Read the model definition and answer for the solid it produces. Units are mm, in the model's axes. Face numbers are marked on the shaded views. A direction names the side the tool comes from. Coordinates: 2 decimals unless noted, no trailing zeros. Loops run counter-clockwise (first coordinate to the right, second up) from the corner with the lowest first, then second, coordinate; pieces in that order, holes last. Notation, with made-up numbers: M -37.5,56.5 L -20.5,56.5 A34 cw -20.5,95.5 Z; hole C -35.5,69 d7. An arc over 180 degrees is marked long. One line per item, written item: value. Start each with the question number.
1. For the marked faces 1, 2, 3 and 4, determine the directions among +Z, -Z, +X, -X, +Y, -Y from which every point of the face is accessible in a straight line to the end or side of a thin tool.
2. Flat-ended cylindrical pins translate along their axes: pin 1 (6.5 mm diameter, centred on x = 98, z = 13.5, fed in from +Y); pin 2 (6.5 mm diameter, centred on y = -7, z = 27, fed in from +X); pin 3 (2 mm diameter, centred on y = -10, z = 28.5, fed in from -X). Find the tip coordinate at first contact, or state that the pin passes through.
3. The part is cut by section B-B (z = 20.3). Write down the section's boundary in (x, y), then the cut area to 3 significant figures.
4. The part is cut by section A-A (y = -13.5). Write down the section's boundary in (x, z), then the cut area to 3 significant figures.
5. Consider probe 1 along X at (y, z) = (-5.7, 20.3); probe 2 along X at (y, z) = (-7.75, 30); probe 3 along X at (y, z) = (-12.25, 17.5). Determine where each line is inside the solid, lowest interval first.
6. The part is cut by section D-D (z = 7.3). Write down the section's boundary in (x, y), then the cut area to 3 significant figures.
7. The part is cut by section C-C (x = 53). Write down the section's boundary in (y, z), then the cut area to 3 significant figures.
```python
from build123d import *

# Parameters (mm, degrees)
BOSS_EXTRUDE1_DEPTH = 40.6
SKETCH2_R           = 1.5
CUT_EXTRUDE3_DEPTH  = 24
SKETCH5_R           = 1.5
CUT_EXTRUDE4_DEPTH  = 4


with BuildPart() as part:
    # Sketch1 → Boss-Extrude1 (new body)
    with BuildSketch(Plane.XY):
        Polygon((8.125196993, -3.6), (8.125196993, -11.6), (0.125196993, -11.6), (0.125196993, -14.6), (11.125196993, -14.6), (11.125196993, -6.6), (89.125196993, -6.6), (89.125196993, -14.6), (100.125196993, -14.6), (100.125196993, -11.6), (92.125196993, -11.6), (92.125196993, -3.6), align=None)
    extrude(amount=BOSS_EXTRUDE1_DEPTH)

    # Sketch2 → Cut-Extrude3 (cut)
    with BuildSketch(Plane.XZ.offset(14.6)):
        with BuildLine():
            Line((89.125196993, 0.154767421), (89.125196993, 0))
            Line((89.125196993, 0), (100.125196993, 0))
            Line((100.125196993, 0), (100.125196993, 13))
            ThreePointArc((100.125196993, 13), (96.999405822, 4.544232737), (89.125196993, 0.154767421))
        make_face()
        with BuildLine():
            Line((89.125196993, 40.6), (89.125196993, 40.445232579))
            ThreePointArc((89.125196993, 40.445232579), (96.999405822, 36.055767263), (100.125196993, 27.6))
            Line((100.125196993, 27.6), (100.125196993, 40.6))
            Line((100.125196993, 40.6), (89.125196993, 40.6))
        make_face()
        with BuildLine():
            Line((0.125196993, 0), (11.125196993, 0))
            Line((11.125196993, 0), (11.125196993, 0.154767421))
            ThreePointArc((11.125196993, 0.154767421), (3.250988164, 4.544232737), (0.125196993, 13))
            Line((0.125196993, 13), (0.125196993, 0))
        make_face()
        with BuildLine():
            ThreePointArc((0.125196993, 27.6), (3.250988164, 36.055767263), (11.125196993, 40.445232579))
            Line((11.125196993, 40.445232579), (11.125196993, 40.6))
            Line((11.125196993, 40.6), (0.125196993, 40.6))
            Line((0.125196993, 40.6), (0.125196993, 27.6))
        make_face()
        with Locations((94.325196993, 33.3)):
            Circle(SKETCH2_R)
        with Locations((94.325196993, 7.3)):
            Circle(SKETCH2_R)
        with Locations((5.925196993, 33.3)):
            Circle(SKETCH2_R)
        with Locations((5.925196993, 7.3)):
            Circle(SKETCH2_R)
    extrude(amount=-CUT_EXTRUDE3_DEPTH, mode=Mode.SUBTRACT)

    # Sketch5 → Cut-Extrude4 (cut)
    with BuildSketch(Plane(origin=(0, -3.6, 0), x_dir=(1, 0, 0), z_dir=(0, 1, 0))):
        with Locations((25.425196993, -20.3)):
            Circle(SKETCH5_R)
        with Locations((74.825196993, -20.3)):
            Circle(SKETCH5_R)
    extrude(amount=-CUT_EXTRUDE4_DEPTH, mode=Mode.SUBTRACT)


solid = part.part
```
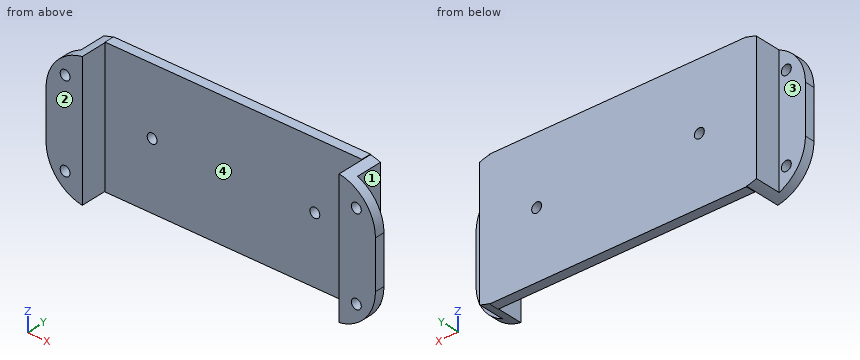
Answer block:
1. face 1: +Z, -Z, +X, +Y
1. face 2: +Z, -Z, +X, -X, -Y
1. face 3: +Z, -Z, -X, +Y
1. face 4: +Z, -Z, -Y
2. pin 1: stops at y = -11.6
2. pin 2: stops at x = 92.13
2. pin 3: stops at x = 8.13
3. outline: M 0.13,-14.6 L 11.13,-14.6 L 11.13,-6.6 L 23.93,-6.6 L 23.93,-3.6 L 8.13,-3.6 L 8.13,-11.6 L 0.13,-11.6 Z; M 26.93,-6.6 L 73.33,-6.6 L 73.33,-3.6 L 26.93,-3.6 Z; M 76.33,-6.6 L 89.13,-6.6 L 89.13,-14.6 L 100.13,-14.6 L 100.13,-11.6 L 92.13,-11.6 L 92.13,-3.6 L 76.33,-3.6 Z
3. area: 330 mm2
4. outline: M 0.13,13 A13 ccw 11.13,0.15 L 11.13,40.45 A13 ccw 0.13,27.6 Z; M 89.13,0.15 A13 ccw 100.13,13 L 100.13,27.6 A13 ccw 89.13,40.45 Z; hole C 5.93,7.3 d3; hole C 5.93,33.3 d3; hole C 94.33,7.3 d3; hole C 94.33,33.3 d3
4. area: 720 mm2
5. probe 1: x = 8.13 to 23.93, 26.93 to 73.33, 76.33 to 92.13
5. probe 2: x = 8.13 to 11.13, 89.13 to 92.13
5. probe 3: x = 0.13 to 11.13, 89.13 to 100.13
6. outline: M 1.44,-14.6 L 4.43,-14.6 L 4.43,-11.6 L 1.44,-11.6 Z; M 7.43,-14.6 L 11.13,-14.6 L 11.13,-6.6 L 89.13,-6.6 L 89.13,-14.6 L 92.83,-14.6 L 92.83,-11.6 L 92.13,-11.6 L 92.13,-3.6 L 8.13,-3.6 L 8.13,-11.6 L 7.43,-11.6 Z; M 95.83,-14.6 L 98.81,-14.6 L 98.81,-11.6 L 95.83,-11.6 Z
6. area: 322 mm2
7. outline: M -6.6,0 L -3.6,0 L -3.6,40.6 L -6.6,40.6 Z
7. area: 122 mm2
